```python
from build123d import *

# Parameters (mm, degrees)
SKETCH001_R       = 0.25
PAD001_DEPTH      = 5.25
PAD001_DEPTH_BACK = 3.5
SKETCH_R          = 12.2
SKETCH_R_2        = 2.75
PAD_DEPTH         = 10.5
FILLET_R          = 0.5


with BuildPart() as pad001:
    # Sketch001 → Pad001 (new body, two sides)
    with BuildSketch(Plane.XY.offset(0.5)) as pad001_sk:
        Circle(SKETCH001_R)
        with Locations((22.9, 0)):
            Circle(SKETCH001_R)
    extrude(amount=PAD001_DEPTH)
    extrude(pad001_sk.sketch, amount=-PAD001_DEPTH_BACK)


with BuildPart() as obj1:
    # Sketch → Pad (new body)
    with BuildSketch(Plane.XY.offset(0.1)):
        with Locations((11.45, 0)):
            Circle(SKETCH_R)
        with Locations((11.45, 0)):
            Circle(SKETCH_R_2, mode=Mode.SUBTRACT)
    extrude(amount=PAD_DEPTH)

    # Fillet
    fillet_edges = [obj1.edges().sort_by_distance(p)[0] for p in [
        (8.7, 0, 10.6),
        (-0.75, 0, 10.6),
        (-0.75, 0, 0.1),
    ]]
    fillet(fillet_edges, radius=FILLET_R)

    # obj1: union Pad001
    add(pad001.part)


solid = obj1.part
```
Source: CAD feature listing. Evaluate the final solid. Frame: model axes, mm. Coordinates: 2 decimals unless noted, no trailing zeros. Loops run counter-clockwise (first coordinate to the right, second up) from the corner with the lowest first, then second, coordinate; pieces in that order, holes last. Notation, with made-up numbers: M -34.75,53.25 L 8.25,53.25 A8 ccw 8.25,65.25 Z; hole C -15,-35.5 d10. An arc over 180 degrees is marked long. Use a Markdown table: item, result. Add a question column.
Q1. Material intervals for L1, parallel to Y at x = 11.45, z = 3.75; L2, parallel to X at y = -0.75, z = 7; L3, parallel to Z at x = 12, y = -5.5, sorted ascending.
Q2. First-contact query: pin 1 (2 mm diameter, centred on y = 7.5, z = 1, fed in from +X); pin 2 (2 mm diameter, centred on x = 20, z = 6.5, fed in from +Y); pin 3 (1.5 mm diameter, centred on y = -7, z = -1, fed in from +X); pin 4 (5 mm diameter, centred on x = 2.5, z = 0, fed in from +Y). Flat tips, straight axial feed; report the tip coordinate or a pass-through.
Q3. Section query A-A, the plane x = 11.45. Return loops of the section in (y, z), and give its area (3 significant figures).
Q4. Draft query along Y for faces 1 (the flat face through (11, 3, 0.1)), 2 (the cylindrical face through (13.99, -1.05, 5.03)), 3 (the cylindrical face through (1.768, -7.424, 5.283)). Return one class per face: pulls with the +Y half, pulls with the -Y half, needs draft (parallel to the pull), parting line crosses it, or undercut.
Q5. Section query B-B, the plane z = 1. Return loops of the section in (x, y), and give its area (3 significant figures).
Result:
| question | item | result |
|---|---|---|
| 1 | L1 | y = -12.2 to -2.75, 2.75 to 12.2 |
| 1 | L2 | x = -0.73 to 8.8, 14.1 to 23.63 |
| 1 | L3 | z = 0.1 to 10.6 |
| 2 | pin 1 | stops at x = 21.77 |
| 2 | pin 2 | stops at y = 9.58 |
| 2 | pin 3 | passes through |
| 2 | pin 4 | stops at y = 10.31 |
| 3 | outline | M -12.2,0.6 A0.5 ccw -11.7,0.1 L -2.75,0.1 L -2.75,10.1 A0.5 ccw -3.25,10.6 L -11.7,10.6 A0.5 ccw -12.2,10.1 Z; M 2.75,0.1 L 11.7,0.1 A0.5 ccw 12.2,0.6 L 12.2,10.1 A0.5 ccw 11.7,10.6 L 3.25,10.6 A0.5 ccw 2.75,10.1 Z |
| 3 | area | 198 mm2 |
| 4 | face 1 | needs draft |
| 4 | face 2 | undercut |
| 4 | face 3 | parting line crosses it |
| 5 | outline | C 11.45,0 d24.4; hole C 11.45,0 d5.5 |
| 5 | area | 444 mm2 |
